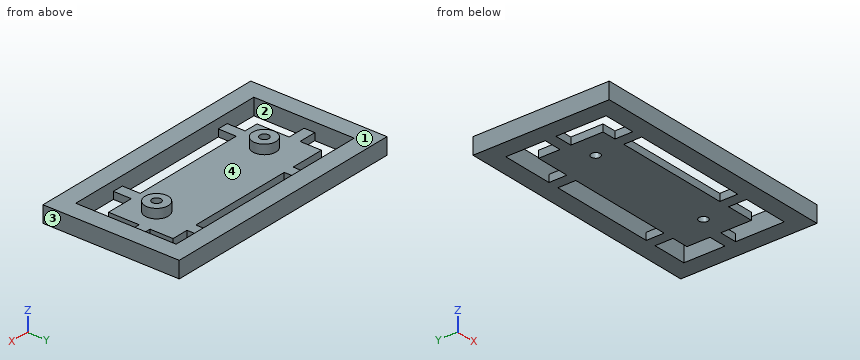
from build123d import *

# Parameters (mm, degrees)
F1_DEPTH  = 2
F2_R      = 3.25
F3_DEPTH  = 2.6
F0_W      = 3
F0_H      = 5
F5_DEPTH  = 2
F6_R      = 1.25
F7_DEPTH  = 25
F8_R      = 1.25
F9_DEPTH  = 25
F0_W_2    = 5
F0_H_2    = 3
F10_DEPTH = 2
F11_DEPTH = 2
F12_DEPTH = 2
F13_DEPTH = 2
F14_W     = 70
F14_H     = 38
F14_W_2   = 60
F14_H_2   = 28
F15_DEPTH = 4.6


# Not quite as in the source:
# - a feature names something its author has since deleted; it is built from what else it names


with BuildPart() as f1:
    # F0 (on Top) → F1 (new body)
    with BuildSketch(Plane.XY):
        Polygon((-13.6037096381, 18), (-23.153355509, 18), (-23.153355509, 12), (-23.153355509, 9), (-23.153355509, 0), (-19.1677454859, 0), (-16.1677454859, 0), (16.1677454859, 0), (19.1677454859, 0), (23.153355509, 0), (26.846644491, 0), (26.846644491, 8.565065451), (26.846644491, 11.565065451), (26.846644491, 18), (22.1654525697, 18), (19.1654525697, 18), (-10.6037096381, 18), align=None)
    extrude(amount=F1_DEPTH)

    # F2 (on face) → F3 (join)
    with BuildSketch(Plane.XY.offset(2)):
        with Locations((19.996644491, 7.75)):
            Circle(F2_R)
        with Locations((-16.303355509, 7.75)):
            Circle(F2_R)
    extrude(amount=F3_DEPTH)

    # F0 (on Top) → F5 (join)
    with BuildSketch(Plane.XY):
        with Locations((20.6654525697, 20.5)):
            Rectangle(F0_W, F0_H)
    extrude(amount=F5_DEPTH)

    # F6 (on face) → F7 (cut)
    with BuildSketch(Plane.XY.offset(4.6)):
        with Locations((-16.303355509, 7.75)):
            Circle(F6_R)
    extrude(amount=-F7_DEPTH, mode=Mode.SUBTRACT)

    # F8 (on face) → F9 (cut)
    with BuildSketch(Plane.XY.offset(4.6)):
        with Locations((19.9292600155, 7.6608564705)):
            Circle(F8_R)
    extrude(amount=-F9_DEPTH, mode=Mode.SUBTRACT)

    # F0 (on Top) → F10 (join)
    with BuildSketch(Plane.XY):
        with Locations((29.346644491, 10.065065451)):
            Rectangle(F0_W_2, F0_H_2)
        with Locations((-25.653355509, 10.5)):
            Rectangle(F0_W_2, F0_H_2)
    extrude(amount=F10_DEPTH)

    # F0 (on Top) → F11 (join)
    with BuildSketch(Plane.XY):
        with Locations((17.6677454859, -2.5)):
            Rectangle(F0_W, F0_H)
    extrude(amount=F11_DEPTH)

    # F0 (on Top) → F12 (join)
    with BuildSketch(Plane.XY):
        with Locations((-17.6677454859, -2.5)):
            Rectangle(F0_W, F0_H)
    extrude(amount=F12_DEPTH)

    # F0 (on Top) → F13 (join)
    with BuildSketch(Plane.XY):
        with Locations((-12.1037096381, 20.5)):
            Rectangle(F0_W, F0_H)
    extrude(amount=F13_DEPTH)

    # F14 (on Top) → F15 (join)
    with BuildSketch(Plane.XY):
        with Locations((1.846644491, 9)):
            Rectangle(F14_W, F14_H)
        with Locations((1.846644491, 9)):
            Rectangle(F14_W_2, F14_H_2, mode=Mode.SUBTRACT)
    extrude(amount=F15_DEPTH)


solid = f1.part
Build history of the part. All positions in model axes, mm. Face numbers are marked on the shaded views. A direction names the side the tool comes from. Coordinates: 2 decimals unless noted, no trailing zeros. Order: outer loops, then holes, each group sorted by start corner. A loop starts at its lowest first (then second) coordinate and runs counter-clockwise, first axis right, second up. Notation, with made-up numbers: (22.5, -33.75) -> (29.5, -33.75) arc R20 ccw to (29.5, -25.75) -> close; hole circle Ø7 at (81, -15). An arc over 180 degrees is marked (long way). One line per item, written item: value.
(1) Tool access for the marked faces 3 and 4: list every direction of +Z, -Z, +X, -X, +Y, -Y with a clear straight run to the whole face (end or side of a thin tool).
Checked values:
face 3: +Z, -Z, +X, +Y, -Y
face 4: +Z
(2) Drop flat-ended pins along their axis: pin 1 Ø8 at (x, y) = (7, 18) entering from -Z; pin 2 Ø8.5 at (x, y) = (11.5, 7.5) entering from +Z. Give the stop position or say it passes through.
Checked values:
pin 1: z = 0
pin 2: z = 2
(3) Slice it at B-B, the plane z = 2.65. List the corners of the cut face in (x, y).
Checked values:
outline: (-33.15, -10) -> (36.85, -10) -> (36.85, 28) -> (-33.15, 28) -> close; circle Ø6.5 at (-16.3, 7.75); circle Ø6.5 at (20, 7.75); hole (-28.15, -5) -> (31.85, -5) -> (31.85, 23) -> (-28.15, 23) -> close; hole circle Ø2.5 at (-16.3, 7.75); hole circle Ø2.5 at (19.93, 7.66)
(4) Slice it at A-A, the plane x = 6. List the corners of the cut face in (y, z), plus the area to 3 significant figures.
Checked values:
outline: (-10, 0) -> (-5, 0) -> (-5, 4.6) -> (-10, 4.6) -> close; (0, 0) -> (18, 0) -> (18, 2) -> (0, 2) -> close; (23, 0) -> (28, 0) -> (28, 4.6) -> (23, 4.6) -> close
area: 82.0 mm2
(5) Slice it at D-D, the plane x = -11.5. List the corners of the cut face in (y, z), plus the area to 3 significant figures.
Checked values:
outline: (-10, 0) -> (-5, 0) -> (-5, 4.6) -> (-10, 4.6) -> close; (0, 0) -> (28, 0) -> (28, 4.6) -> (23, 4.6) -> (23, 2) -> (0, 2) -> close
area: 92.0 mm2
(6) Slice it at C-C, the plane y = 3. List the corners of the cut face in (x, z), plus the area to 3 significant figures.
Checked values:
outline: (-33.15, 0) -> (-28.15, 0) -> (-28.15, 4.6) -> (-33.15, 4.6) -> close; (-23.15, 0) -> (26.85, 0) -> (26.85, 2) -> (-23.15, 2) -> close; (31.85, 0) -> (36.85, 0) -> (36.85, 4.6) -> (31.85, 4.6) -> close
area: 146 mm2
(7) Mould opens along Y. For the marked faces 1 and 2 say: pulls with the +Y half, pulls with the -Y half, needs draft (parallel to the pull), parting line crosses it, or undercut.
Checked values:
face 1: needs draft
face 2: undercut
(8) Probe line 1 (Y direction, x = -22.5, z = 0.6); line 2 (X direction, y = 22, z = 1.05); line 3 (X direction, y = 15.5, z = 1.4). List the from-to ranges inside material, lowest first. Write a range as [from, to].
Checked values:
line 1: [-10, -5], [0, 18], [23, 28]
line 2: [-33.15, -28.15], [-13.6, -10.6], [19.17, 22.17], [31.85, 36.85]
line 3: [-33.15, -28.15], [-23.15, 26.85], [31.85, 36.85]
